Read the model definition and answer for the solid it produces. Units are mm, in the model's axes. Face numbers are marked on the shaded views. A direction names the side the tool comes from. Coordinates: 2 decimals unless noted, no trailing zeros. Order: outer loops, then holes, each group sorted by start corner. A loop starts at its lowest first (then second) coordinate and runs counter-clockwise, first axis right, second up. Notation, with made-up numbers: (69.25, 66) - (74.25, 66) arc R19 ccw to (74.25, 85) - close; hole circle Ø6 at (-15, 6.25). An arc over 180 degrees is marked (long way). Answer as a JSON object with one key per item and string values. Group by question number.
from build123d import *

# Parameters (mm, degrees)
F0_W     = 25.4
F0_H     = 25.4
F1_DEPTH = 12.7
F2_T     = -2.54
F4_DEPTH = 25.401


with BuildPart() as f1:
    # F0 (on Front) → F1 (new body, symmetric)
    with BuildSketch(Plane.XZ):
        Rectangle(F0_W, F0_H)
    extrude(amount=F1_DEPTH, both=True)

    # F2
    f2_openings = [f1.faces().sort_by_distance(p)[0] for p in [
        (0, 0, 12.7),
        (0, 0, -12.7),
    ]]
    offset(amount=F2_T, openings=f2_openings)

    # F3 (on face) → F4 (cut, through all)
    with BuildSketch(Plane.YZ.offset(12.7)):
        Polygon((-12.7, 12.7), (-12.7, 9.525), (12.7, 12.7), align=None)
    extrude(amount=-F4_DEPTH, mode=Mode.SUBTRACT)


solid = f1.part
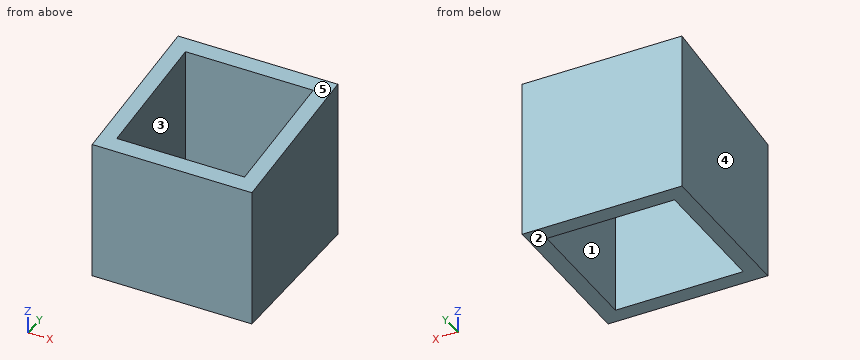
1. Straight lines are drawn through the part: L1, parallel to Y at x = -4, z = 5.5; L2, parallel to Y at x = 4, z = 10. For each, find the intervals that lie inside material, in ascending order.
2. A cutting plane is placed at A-A on x = 2. Write down the section's boundary in (y, z) (1 decimal).
3. For the marked faces 1 and 2, determine the directions among +Z, -Z, +X, -X, +Y, -Y from which every point of the face is accessible in a straight line to the end or side of a thin tool.
4. A cutting plane is placed at C-C on z = -3. Write down the section's boundary in (x, y).
5. A cutting plane is placed at B-B on y = 1.5. Write down the section's boundary in (x, z).
6. For a pull along X with two mould halves and no side action, classify the marked faces 3, 4 and 5 as pulls with the +X half, pulls with the -X half, needs draft (parallel to the pull), parting line crosses it, or undercut.
7. Given pin 1 (1.5 mm diameter, centred on x = -8, y = -2.5, fed in from +Z), flat-ended and moving along its own axis, determine where the tip first touches the part or whether it passes through.
Derived:
{
 "1": {"L1": "y = -12.7 to -10.16, 10.16 to 12.7", "L2": "y = 10.16 to 12.7"},
 "2": {"outline": "(-12.7, -12.7) - (-10.2, -12.7) - (-10.2, 9.8) - (-12.7, 9.5) - close; (10.2, -12.7) - (12.7, -12.7) - (12.7, 12.7) - (10.2, 12.4) - close"},
 "3": {"face 1": "+Z, -Z", "face 2": "-Z, +X, -X, +Y, -Y"},
 "4": {"outline": "(-12.7, -12.7) - (12.7, -12.7) - (12.7, 12.7) - (-12.7, 12.7) - close; hole (-10.16, -10.16) - (10.16, -10.16) - (10.16, 10.16) - (-10.16, 10.16) - close"},
 "5": {"outline": "(-12.7, -12.7) - (-10.16, -12.7) - (-10.16, 11.3) - (-12.7, 11.3) - close; (10.16, -12.7) - (12.7, -12.7) - (12.7, 11.3) - (10.16, 11.3) - close"},
 "6": {"face 3": "undercut", "face 4": "pulls with the -X half", "face 5": "needs draft"},
 "7": {"pin 1": "passes through"}
}
